The model under review builds one solid part; all positions refer to its coordinate system, in mm. Face numbers are marked on the shaded views. A direction names the side the tool comes from. Give positions to 0.01 mm unless a question says otherwise; leave off trailing zeros. Order: outer loops, then holes, each group sorted by start corner. A loop starts at its lowest first (then second) coordinate and runs counter-clockwise, first axis right, second up. Notation, with made-up numbers: (33.25, 82) -> (92.25, 82) arc R33 ccw to (92.25, 113) -> close; hole circle Ø5 at (3, 55.5). An arc over 180 degrees is marked (long way). Answer as a JSON object with one key per item and string values. Group by question number.
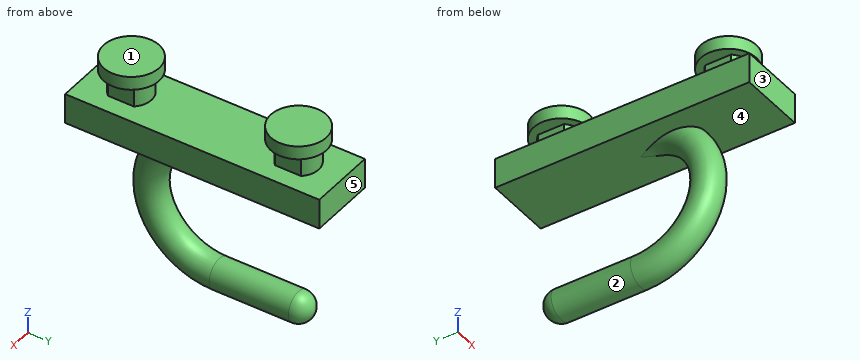
from build123d import *

# Parameters (mm, degrees)
EXTRUDE_1_DEPTH   = 3.5
EXTRUDE_1_2_DEPTH = 3.5
SKETCH_2_R        = 4.15
EXTRUDE_2_DEPTH   = 2
SKETCH_3_W        = 10
SKETCH_3_H        = 38
EXTRUDE_3_DEPTH   = 4.5
SKETCH_5_R        = 2.25


with BuildPart() as part:
    # Sketch 1 → Extrude 1 (new body)
    with BuildSketch(Plane.XY):
        with BuildLine():
            Line((-2.3, 1.926136028), (-2.3, -1.926136028))
            ThreePointArc((-2.3, -1.926136028), (0, -3), (2.3, -1.926136028))
            Line((2.3, -1.926136028), (2.3, 1.926136028))
            ThreePointArc((2.3, 1.926136028), (0, 3), (-2.3, 1.926136028))
        make_face()
    extrude(amount=EXTRUDE_1_DEPTH)



with BuildPart() as body_2:
    # Sketch 1 → Extrude 1 2 (new body)
    with BuildSketch(Plane.XY):
        with BuildLine():
            Line((-2.3, -23.073863972), (-2.3, -26.926136028))
            ThreePointArc((-2.3, -26.926136028), (0, -28), (2.3, -26.926136028))
            Line((2.3, -26.926136028), (2.3, -23.073863972))
            ThreePointArc((2.3, -23.073863972), (0, -22), (-2.3, -23.073863972))
        make_face()
    extrude(amount=EXTRUDE_1_2_DEPTH)


with BuildPart() as part_1:
    add(part.part)

    add(body_2.part)  # Extrude 2 merges body 2
    # Sketch 2 → Extrude 2 (add)
    with BuildSketch(Plane.XY.offset(3.5)):
        Circle(SKETCH_2_R)
        with Locations((0, -25)):
            Circle(SKETCH_2_R)
    extrude(amount=EXTRUDE_2_DEPTH)

    # Sketch 3 → Extrude 3 (add)
    with BuildSketch(Plane(origin=(0, 0, 0), x_dir=(-1, 0, 0), z_dir=(0, 0, -1))):
        with Locations((0, -12.5)):
            Rectangle(SKETCH_3_W, SKETCH_3_H)
    extrude(amount=EXTRUDE_3_DEPTH)

    # Sweep 1: sweep along a path in Sketch 4
    with BuildLine(Plane(origin=(0, 0, 0), x_dir=(0, 0, -1), z_dir=(1, 0, 0))) as sweep_1_path:
        Line((2.25, 0), (2.25, -11.85))
        ThreePointArc((2.25, -11.85), (12.4, -22), (22.55, -11.85))
        Line((22.55, -11.85), (22.55, 0))
    # Sketch 5 → Sweep 1 (sweep)
    with BuildSketch(Plane(origin=(0, 0, 0), x_dir=(1, 0, 0), z_dir=(0, 1, 0))):
        with Locations((0, 22.55)):
            Circle(SKETCH_5_R)
    sweep(path=sweep_1_path.line)

    # Sketch 6 → Revolve 1 (revolve)
    with BuildSketch(Plane(origin=(0, 0, 0), x_dir=(0, 0, -1), z_dir=(1, 0, 0))):
        with BuildLine():
            Line((22.55, 0), (22.55, 2.25))
            ThreePointArc((22.55, 2.25), (20.959009742, 1.590990258), (20.3, 0))
            Line((20.3, 0), (22.55, 0))
        make_face()
    revolve(axis=Axis((0, 0, -22.55), (0, 1, 0)))


solid = part_1.part
1. For pin 1 (1.8 mm diameter, centred on y = -24, z = 1, fed in from -X); pin 2 (6 mm diameter, centred on x = -2, y = -16.5, fed in from +Z); pin 3 (1.5 mm diameter, centred on y = -2.5, z = -6, fed in from -X); pin 4 (1.5 mm diameter, centred on x = 1, y = -16.5, fed in from -Z), all flat-tipped, find the tip position at first contact; note any pin that passes through.
2. Draft analysis for pull direction Z (two halves, no side actions). For the marked faces 1, 2 and 3, state which applies: pulls with the +Z half, pulls with the -Z half, needs draft (parallel to the pull), parting line crosses it, or undercut.
3. Machinability: for the marked faces 4 and 5, which of the approach directions +Z, -Z, +X, -X, +Y, -Y give a long, thin tool a straight path to every point of the face, cutting with its end or side? Answer none if there is none.
4. Take a section at A-A on x = -2.75. Give the boundary of the cut face in (y, z).
5. Take a section at B-B on x = 0.5. Give the boundary of the cut face in (y, z), plus the area to 3 significant figures.
6. For probe 1 along Z at (x, y) = (2.5, 3); probe 2 along Z at (x, y) = (-4.5, -17); probe 3 along Z at (x, y) = (-0.5, -24.5), list the stretches that pass through material, from the lowest coordinate up. Write a range as [from, to].
Checks:
{
 "1": {"pin 1": "stops at x = -2.3", "pin 2": "stops at z = 0", "pin 3": "passes through", "pin 4": "stops at z = -24.05"},
 "2": {"face 1": "pulls with the +Z half", "face 2": "undercut", "face 3": "needs draft"},
 "3": {"face 4": "none", "face 5": "+Z, -Z, +X, -X, +Y"},
 "4": {"outline": "(-31.5, -4.5) -> (6.5, -4.5) -> (6.5, 0) -> (-31.5, 0) -> close; (-28.11, 3.5) -> (-21.89, 3.5) -> (-21.89, 5.5) -> (-28.11, 5.5) -> close; (-3.11, 3.5) -> (3.11, 3.5) -> (3.11, 5.5) -> (-3.11, 5.5) -> close"},
 "5": {"outline": "(-31.5, -4.5) -> (-21.33, -4.5) arc R12.34 ccw to (-11.85, -24.74) -> (0, -24.74) arc R2.19 ccw to (0, -20.36) -> (-11.85, -20.36) arc R7.96 cw to (-12.79, -4.5) -> (6.5, -4.5) -> (6.5, 0) -> (2.96, 0) -> (2.96, 3.5) -> (4.12, 3.5) -> (4.12, 5.5) -> (-4.12, 5.5) -> (-4.12, 3.5) -> (-2.96, 3.5) -> (-2.96, 0) -> (-22.04, 0) -> (-22.04, 3.5) -> (-20.88, 3.5) -> (-20.88, 5.5) -> (-29.12, 5.5) -> (-29.12, 3.5) -> (-27.96, 3.5) -> (-27.96, 0) -> (-31.5, 0) -> close", "area": "416 mm2"},
 "6": {"probe 1": "z = [-4.5, 0], [3.5, 5.5]", "probe 2": "z = [-4.5, 0]", "probe 3": "z = [-4.5, 5.5]"}
}
